from build123d import *

# Parameters (mm, degrees)
SKETCH1_W           = 80
SKETCH1_H           = 140
BOSS_EXTRUDE1_DEPTH = 2
SKETCH4_W           = 140
SKETCH4_H           = 2
BOSS_EXTRUDE2_DEPTH = 35
SKETCH5_W           = 140
SKETCH5_H           = 2
BOSS_EXTRUDE3_DEPTH = 20
SKETCH2_R           = 2.5
CUT_EXTRUDE1_DEPTH  = 10
SKETCH7_W           = 140
SKETCH7_H           = 2
BOSS_EXTRUDE5_DEPTH = 20
SKETCH8_R           = 2.75
CUT_EXTRUDE2_DEPTH  = 10
SKETCH9_W           = 50
SKETCH9_H           = 2
BOSS_EXTRUDE6_DEPTH = 50
SKETCH10_R          = 2
CUT_EXTRUDE3_DEPTH  = 40
CUT_EXTRUDE4_DEPTH  = 40
CHAMFER1_SIZE       = 49.985180236
CHAMFER1_SIZE_2     = 35
SKETCH12_W          = 60
SKETCH12_H          = 27.596233816
CUT_EXTRUDE5_DEPTH  = 10
CUT_EXTRUDE6_DEPTH  = 10
SKETCH14_W          = 110
SKETCH14_H          = 20
CUT_EXTRUDE7_DEPTH  = 10
FILLET1_R           = 10


# Some blends are built 0.0001 mm under size
with BuildPart() as part:
    # Sketch1 → Boss-Extrude1 (new body)
    with BuildSketch(Plane(origin=(0, 0, 0), x_dir=(1, 0, 0), z_dir=(0, 1, 0))):
        with Locations((40, 70)):
            Rectangle(SKETCH1_W, SKETCH1_H)
    extrude(amount=BOSS_EXTRUDE1_DEPTH)

    # Sketch4 → Boss-Extrude2 (add)
    with BuildSketch(Plane(origin=(80, 0, 0), x_dir=(0, 0, -1), z_dir=(1, 0, 0))):
        with Locations((70, 1)):
            Rectangle(SKETCH4_W, SKETCH4_H)
    extrude(amount=BOSS_EXTRUDE2_DEPTH)

    # Sketch5 → Boss-Extrude3 (add)
    with BuildSketch(Plane(origin=(115, 0, 0), x_dir=(0, 0, -1), z_dir=(1, 0, 0))):
        with Locations((70, 1)):
            Rectangle(SKETCH5_W, SKETCH5_H)
    extrude(amount=BOSS_EXTRUDE3_DEPTH)

    # Sketch2 → Cut-Extrude1 (cut)
    with BuildSketch(Plane.XZ):
        with Locations(Location((97.5, -100, 0), (0, 0, 270))):
            Circle(SKETCH2_R)
        with Locations(Location((97.5, -40, 0), (0, 0, 270))):
            Circle(SKETCH2_R)
        with Locations(Location((37.5, -40, 0), (0, 0, 270))):
            Circle(SKETCH2_R)
        with Locations(Location((37.5, -100, 0), (0, 0, 270))):
            Circle(SKETCH2_R)
    extrude(amount=-CUT_EXTRUDE1_DEPTH, mode=Mode.SUBTRACT)

    # Sketch7 → Boss-Extrude5 (add)
    with BuildSketch(Plane.ZY):
        with Locations((-70, 1)):
            Rectangle(SKETCH7_W, SKETCH7_H)
    extrude(amount=BOSS_EXTRUDE5_DEPTH)

    # Sketch8 → Cut-Extrude2 (cut)
    with BuildSketch(Plane.XZ):
        with Locations(Location((125, -17.5, 0), (0, 0, 270))):
            Circle(SKETCH8_R)
        with Locations(Location((125, -49.5, 0), (0, 0, 270))):
            Circle(SKETCH8_R)
        with Locations(Location((125, -90.5, 0), (0, 0, 270))):
            Circle(SKETCH8_R)
        with Locations(Location((125, -122.5, 0), (0, 0, 270))):
            Circle(SKETCH8_R)
        with Locations(Location((-10, -122.5, 0), (0, 0, 90))):
            Circle(SKETCH8_R)
        with Locations(Location((-10, -90.5, 0), (0, 0, 90))):
            Circle(SKETCH8_R)
        with Locations(Location((-10, -49.5, 0), (0, 0, 90))):
            Circle(SKETCH8_R)
        with Locations(Location((-10, -17.5, 0), (0, 0, 90))):
            Circle(SKETCH8_R)
    extrude(amount=-CUT_EXTRUDE2_DEPTH, mode=Mode.SUBTRACT)

    # Sketch9 → Boss-Extrude6 (add)
    with BuildSketch(Plane(origin=(135, 0, 0), x_dir=(0, 0, -1), z_dir=(1, 0, 0))):
        with Locations((70, 1)):
            Rectangle(SKETCH9_W, SKETCH9_H)
    extrude(amount=BOSS_EXTRUDE6_DEPTH)

    # Sketch10 → Cut-Extrude3 (cut)
    with BuildSketch(Plane.XZ):
        with Locations(Location((175, -55, 0), (0, 0, 270))):
            Circle(SKETCH10_R)
        with Locations(Location((175, -85, 0), (0, 0, 270))):
            Circle(SKETCH10_R)
        with Locations(Location((155, -85, 0), (0, 0, 270))):
            Circle(SKETCH10_R)
        with Locations(Location((155, -55, 0), (0, 0, 270))):
            Circle(SKETCH10_R)
    extrude(amount=-CUT_EXTRUDE3_DEPTH, mode=Mode.SUBTRACT)

    # Sketch11 → Cut-Extrude4 (cut)
    with BuildSketch(Plane.XZ):
        Polygon((135, -11.201883092), (22.258688724, -11.201883092), (-20, -11.201883092), (-20, 0), (135, 0), align=None)
        Polygon((135, -140), (135, -128.798116908), (22.258688724, -128.798116908), (-20, -128.798116908), (-20, -140), align=None)
    extrude(amount=-CUT_EXTRUDE4_DEPTH, mode=Mode.SUBTRACT)

    # Chamfer1
    # the kernel refuses this chamfer: 49.985180236, 35 mm, written as the material it adds along each edge
    with BuildSketch(Plane(origin=(135, 2, -95), x_dir=(0.9997533347641299, 0, 0.022209674198457038), z_dir=(0, -1, 0))) as chamfer1_piece_1_section:
        Polygon((CHAMFER1_SIZE * 0.999753334764, -CHAMFER1_SIZE * 0.0222096741984), (-CHAMFER1_SIZE_2 * 0.0222096741985, -CHAMFER1_SIZE_2 * 0.999753334764), (0, 0), align=None)
    chamfer1_piece_1 = extrude(amount=2, mode=Mode.PRIVATE)
    chamfer1_piece_1 = split(chamfer1_piece_1, bisect_by=Plane(origin=(151.760683993, 1, -128.798116908), z_dir=(0, 0, 1)), keep=Keep.TOP, mode=Mode.PRIVATE)
    add(chamfer1_piece_1)
    with BuildSketch(Plane(origin=(135, 0, -45), x_dir=(-0.045263737714021514, 0, 0.9989750717851553), z_dir=(0, 1, 0))) as chamfer1_piece_2_section:
        Polygon((CHAMFER1_SIZE_2 * 0.998975071785, CHAMFER1_SIZE_2 * 0.045263737714), (-CHAMFER1_SIZE * 0.045263737714, CHAMFER1_SIZE * 0.998975071785), (0, 0), align=None)
    chamfer1_piece_2 = extrude(amount=2, mode=Mode.PRIVATE)
    chamfer1_piece_2 = split(chamfer1_piece_2, bisect_by=Plane(origin=(151.760683993, 1, -11.201883092), z_dir=(0, 0, -1)), keep=Keep.TOP, mode=Mode.PRIVATE)
    add(chamfer1_piece_2)

    # Sketch12 → Cut-Extrude5 (cut)
    with BuildSketch(Plane.XZ):
        with Locations((10, -70)):
            Rectangle(SKETCH12_W, SKETCH12_H)
    extrude(amount=-CUT_EXTRUDE5_DEPTH, mode=Mode.SUBTRACT)

    # Sketch13 → Cut-Extrude6 (cut)
    with BuildSketch(Plane.XZ):
        Polygon((184.985180236, -45), (136.716466943, -45), (136.716466943, -11.201883092), align=None)
        Polygon((184.985180236, -95), (136.716466943, -128.798116908), (136.716466943, -95), align=None)
    extrude(amount=-CUT_EXTRUDE6_DEPTH, mode=Mode.SUBTRACT)

    # Sketch14 → Cut-Extrude7 (cut)
    with BuildSketch(Plane.XZ):
        with Locations((60, -21.201883092)):
            Rectangle(SKETCH14_W, SKETCH14_H)
        with Locations((60, -118.798116908)):
            Rectangle(SKETCH14_W, SKETCH14_H)
    extrude(amount=-CUT_EXTRUDE7_DEPTH, mode=Mode.SUBTRACT)

    # Fillet1
    fillet1_edges = [part.edges().sort_by_distance(p)[0] for p in [
        (185, 1, -45),
        (185, 1, -95),
        (-20, 1, -128.798116908),
        (-20, 1, -11.201883092),
        (136.716466943, 1, -128.798116908),
        (136.716466943, 1, -11.201883092),
        (-20, 1, -83.798116908),
        (-20, 1, -56.201883092),
        (40, 1, -56.201883092),
        (40, 1, -83.798116908),
        (136.716466943, 1, -45),
        (136.716466943, 1, -95),
        (115, 1, -11.201883092),
        (5, 1, -11.201883092),
        (5, 1, -128.798116908),
        (115, 1, -128.798116908),
        (5, 1, -31.201883092),
        (115, 1, -31.201883092),
        (115, 1, -108.798116908),
        (5, 1, -108.798116908),
    ]]
    fillet(fillet1_edges, radius=FILLET1_R - 0.0001)  # a hair under: the kernel refuses the full size


solid = part.part
Read the model definition and answer for the solid it produces. Units are mm, in the model's axes. A direction names the side the tool comes from. Give positions to 0.01 mm unless a question says otherwise; leave off trailing zeros. Write each loop counter-clockwise with the first axis right and the second up, starting at its lowest first coordinate (ties: lowest second). Pieces come first, ordered by that corner, then holes. Notation, with made-up numbers: (87, 26.25) -> (138, 26.25) arc R12 ccw to (138, 46.25) -> close; hole circle Ø7 at (-34, 73). An arc over 180 degrees is marked (long way). Answer as a JSON object with one key per item and string values. Group by question number.
1) Find section D-D (y = 1.3). Count the separate pieces of the cut face and the enclosed holes in it, and give its area (3 significant figures).
2) Find section A-A (x = 17.5). Write down the section's boundary in (y, z), and give its area (3 significant figures).
3) Consider L1, parallel to Z at x = -10, y = 0.7; L2, parallel to Z at x = 175, y = 1.4; L3, parallel to X at y = 0.5, z = -55. Determine where each line is inside the solid, lowest interval first. Write a range as from..to.
4) A tool of negligible diameter and unlimited length cuts with its end or side. For faces 4 (the cylindrical face through (182.15, 1.01, -91.99)), 5 (the cylindrical face through (118.01, 1.01, -14.05)), 6 (the cylindrical face through (37.15, 1.01, -80.79)), 7 (the cylindrical face through (1.99, 1.01, -125.95)), from which of +Z, -Z, +X, -X, +Y, -Y can it reach the whole face along a straight path? Write none if from no direction.
5) Find section B-B (z = -49.5). Write down the section's boundary in (x, y).
6) The mould has two halves that part along Z. Classify faces 1 (the cylindrical face through (181.99, 1.01, -47.85)), 2 (the flat face through (83, 0, -70)), 3 (the cylindrical face through (123.327, 0.986, -88.318)): +Z half, -Z half, draft (parallel to the pull), parting line (faces both ways), or undercut.
7) Find section C-C (z = -122.5). Write down the section's boundary in (x, y), and give its area (3 significant figures).
8) Each of these flat-tipped pins is pushed along its axis until it touches: P1, Ø0.6, axis at y = 1, z = -112.5, coming from the +X side; P2, Ø6.5, axis at x = 37.5, z = -40, coming from the +Y side; P3, Ø5, axis at x = 125, z = -49.5, coming from the -Y side; P4, Ø0.6, axis at x = 162, y = 0.5, coming from the -Z side. Where does it stop, or does it pass through?
Values follow:
{
 "1": {"separate pieces": "1", "enclosed holes": "16", "area": "14,400 mm2"},
 "2": {"outline": "(0, -108.8) -> (2, -108.8) -> (2, -83.8) -> (0, -83.8) -> close; (0, -56.2) -> (2, -56.2) -> (2, -31.2) -> (0, -31.2) -> close", "area": "100 mm2"},
 "3": {"L1": "z = -128.8..-125.25, -119.75..-93.25, -87.75..-83.8, -56.2..-52.25, -46.75..-20.25, -14.75..-11.2", "L2": "z = -95..-87, -83..-57, -53..-45", "L3": "x = -14.75..153, 157..173, 177..185"},
 "4": {"face 4": "-Z, +X, +Y, -Y", "face 5": "+Z, +Y, -Y", "face 6": "-X, +Y, -Y", "face 7": "-Z, +Y, -Y"},
 "5": {"outline": "(-19.44, 0) -> (-12.75, 0) -> (-12.75, 2) -> (-19.44, 2) -> close; (-7.25, 0) -> (122.25, 0) -> (122.25, 2) -> (-7.25, 2) -> close; (127.75, 0) -> (183.35, 0) -> (183.35, 2) -> (127.75, 2) -> close"},
 "6": {"face 1": "+Z half", "face 2": "draft", "face 3": "undercut"},
 "7": {"outline": "(-19.29, 0) -> (-12.75, 0) -> (-12.75, 2) -> (-19.29, 2) -> close; (-7.25, 0) -> (4.29, 0) -> (4.29, 2) -> (-7.25, 2) -> close; (115.71, 0) -> (122.25, 0) -> (122.25, 2) -> (115.71, 2) -> close; (127.75, 0) -> (136.01, 0) -> (136.01, 2) -> (127.75, 2) -> close", "area": "65.7 mm2"},
 "8": {"P1": "stops at x = 136.72", "P2": "stops at y = 2", "P3": "passes through", "P4": "stops at z = -95"}
}
